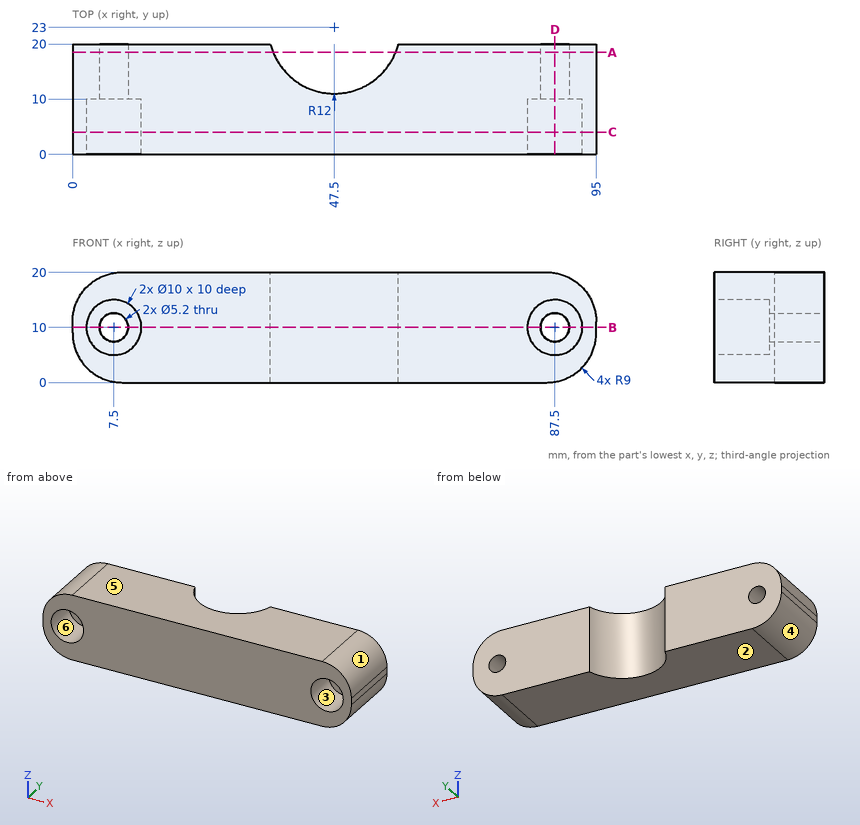
Can you work these out from the drawing? Everything is in mm from the part's minimum corner. A direction names the side the tool comes from. Give positions to 0.01 mm unless a question says otherwise; leave off trailing zeros. Loops run counter-clockwise (first coordinate to the right, second up) from the corner with the lowest first, then second, coordinate; pieces in that order, holes last. Notation, with made-up numbers: (32, 36) -> (69, 36) arc R23 cw to (69, 58) -> close; hole circle Ø9 at (13.25, -12). An arc over 180 degrees is marked (long way). Return JSON: item names as keys, results as strings.
Q1. I want a section at B-B, the plane z = 10. List the corners of the cut face in (x, y) for me.
Checks:
{"outline": "(0, 0) -> (2.5, 0) -> (2.5, 10) -> (4.9, 10) -> (4.9, 20) -> (0, 20) -> close; (10.1, 10) -> (12.5, 10) -> (12.5, 0) -> (82.5, 0) -> (82.5, 10) -> (84.9, 10) -> (84.9, 20) -> (59.12, 20) arc R12 cw to (35.88, 20) -> (10.1, 20) -> close; (90.1, 10) -> (92.5, 10) -> (92.5, 0) -> (95, 0) -> (95, 20) -> (90.1, 20) -> close"}
Q2. We'd pull the mould along X, two halves only. Please class the marked faces 1, 2, 3 and 4: released by +X, released by -X, zero draft, split by the parting line, or undercut.
Checks:
{"face 1": "released by +X", "face 2": "zero draft", "face 3": "undercut", "face 4": "released by -X"}
Q3. For pin 1 Ø6 at (x, z) = (53.5, 16) entering from +Y; pin 2 Ø3 at (x, z) = (48, 5.5) entering from +Y; pin 3 Ø1.5 at (y, z) = (16.5, 7.5) entering from -X, each with a flat end and sliding along its axis, tell me the tip position at first contact or that it passes through.
Checks:
{"pin 1": "stops at y = 15.06", "pin 2": "stops at y = 11.17", "pin 3": "stops at x = 0.03"}
Q4. On a 3-axis mill with a long thin cutter (end or side, diameter ignored), from which of +Z, -Z, +X, -X, +Y, -Y can I reach the whole of each face in a straight line? I mean the marked faces 5 and 6. Say none if no direction works.
Checks:
{"face 5": "+Z, +X, -X, +Y, -Y", "face 6": "-Y"}
Q5. I need wall thicknesses on probe 1 along X at (y, z) = (1.25, 14); probe 2 along X at (y, z) = (7.5, 11.5); probe 3 along Y at (x, z) = (86, 6). Which ranges of each line are inside material? Lowest first, please.
Checks:
{"probe 1": "x = 0.51 to 4.5, 10.5 to 84.5, 90.5 to 94.49", "probe 2": "x = 0.01 to 2.73, 12.27 to 82.73, 92.27 to 94.99", "probe 3": "y = 10 to 20"}
Q6. I want a section at A-A, the plane y = 18.5. List the corners of the cut face in (x, z) for me.
Checks:
{"outline": "(0, 9) arc R9 ccw to (9, 0) -> (36.38, 0) -> (36.38, 20) -> (9, 20) arc R9 ccw to (0, 11) -> close; (58.62, 0) -> (86, 0) arc R9 ccw to (95, 9) -> (95, 11) arc R9 ccw to (86, 20) -> (58.62, 20) -> close; hole circle Ø5.2 at (7.5, 10); hole circle Ø5.2 at (87.5, 10)"}
Q7. I want a section at D-D, the plane x = 87.5. List the corners of the cut face in (y, z) for me, then the cut area to 3 significant figures.
Checks:
{"outline": "(0, 0.13) -> (20, 0.13) -> (20, 7.4) -> (10, 7.4) -> (10, 5) -> (0, 5) -> close; (0, 15) -> (10, 15) -> (10, 12.6) -> (20, 12.6) -> (20, 19.87) -> (0, 19.87) -> close", "area": "243 mm2"}
Q8. I want a section at C-C, the plane y = 4. List the corners of the cut face in (x, z) for me, then the cut area to 3 significant figures.
Checks:
{"outline": "(0, 9) arc R9 ccw to (9, 0) -> (86, 0) arc R9 ccw to (95, 9) -> (95, 11) arc R9 ccw to (86, 20) -> (9, 20) arc R9 ccw to (0, 11) -> close; hole circle Ø10 at (7.5, 10); hole circle Ø10 at (87.5, 10)", "area": "1,670 mm2"}
